The model under review builds one solid part; all positions refer to its coordinate system, in mm. Give positions to 0.01 mm unless a question says otherwise; leave off trailing zeros. Loops run counter-clockwise (first coordinate to the right, second up) from the corner with the lowest first, then second, coordinate; pieces in that order, holes last. Notation, with made-up numbers: M 78.25,19.25 L 112.25,19.25 A23 ccw 112.25,49.25 Z; hole C 66,22 d11. An arc over 180 degrees is marked long. Put each result on its own line as item: value. Start each with the question number.
from build123d import *

# Parameters (mm, degrees)
SKETCH1_W           = 355.6
SKETCH1_H           = 355.6
BOSS_EXTRUDE1_DEPTH = 9.525
CHAMFER1_SIZE       = 19.05
SKETCH2_W           = 6.35
SKETCH2_H           = 19.05
CUT_EXTRUDE1_DEPTH  = 3.175


with BuildPart() as part:
    # Sketch1 → Boss-Extrude1 (new, symmetric)
    with BuildSketch(Plane(origin=(0, 0, 0), x_dir=(1, 0, 0), z_dir=(0, 1, 0))):
        Rectangle(SKETCH1_W, SKETCH1_H)
    extrude(amount=BOSS_EXTRUDE1_DEPTH, both=True)

    # Chamfer1
    chamfer1_edges = [part.edges().sort_by_distance(p)[0] for p in [
        (177.8, -9.525, 0),
        (-177.8, -9.525, 0),
    ]]
    chamfer(chamfer1_edges, length=CHAMFER1_SIZE - 0.0001)  # a hair under: the kernel refuses the full size

    # Sketch2 → Cut-Extrude1 (cut)
    with BuildSketch(Plane.XY.offset(177.8)):
        with Locations((22.225, 0)):
            Rectangle(SKETCH2_W, SKETCH2_H)
        with Locations((-22.225, 0)):
            Rectangle(SKETCH2_W, SKETCH2_H)
    extrude(amount=-CUT_EXTRUDE1_DEPTH, mode=Mode.SUBTRACT)


solid = part.part
(1) To check wall thickness, follow L1, parallel to X at y = -7.5, z = -87; L2, parallel to X at y = 5, z = -22. State the ranges of each line that lie inside material, in increasing order. Write a range as [from, to].
(2) We need section B-B, the plane y = -1.5. Write out the cut boundary in (x, z) (3 decimals).
(3) Draft analysis for pull direction X (two halves, no side actions). For faces 1 (the flat face through (168.142, -0.133, 2.489)), 2 (the flat face through (-2, 0, -177.8)), 3 (the flat face through (-168.142, -0.133, 2.489)), state which applies: +X half, -X half, draft (parallel to the pull), parting line (faces both ways), or undercut.
(4) Insertion check: pin 1 (1.5 mm diameter, centred on y = -3, z = 46, fed in from +X); pin 2 (3 mm diameter, centred on x = 23, y = 1, fed in from +Z) (3 decimals); pin 3 (1.6 mm diameter, centred on y = -1, z = 177, fed in from +X). Each pin has a flat end and moves straight along its axis. Give the tip position at first contact, or say it passes through.
Check sheet entries:
1. L1: x = [-160.78, 160.78]
1. L2: x = [-173.28, 173.28]
2. outline: M -166.775,-177.8 L 166.775,-177.8 L 166.775,177.8 L 25.4,177.8 L 25.4,174.625 L 19.05,174.625 L 19.05,177.8 L -19.05,177.8 L -19.05,174.625 L -25.4,174.625 L -25.4,177.8 L -166.775,177.8 Z
3. face 1: +X half
3. face 2: draft
3. face 3: -X half
4. pin 1: stops at x = 166.03
4. pin 2: stops at z = 174.625
4. pin 3: stops at x = 168.08
